Input: dimensioned drawing with shaded views. Units: mm. Origin: part minimum x, y, z. A direction names the side the tool comes from. Give positions to 0.01 mm unless a question says otherwise; leave off trailing zeros. Write each loop counter-clockwise with the first axis right and the second up, starting at its lowest first coordinate (ties: lowest second). Pieces come first, ordered by that corner, then holes.
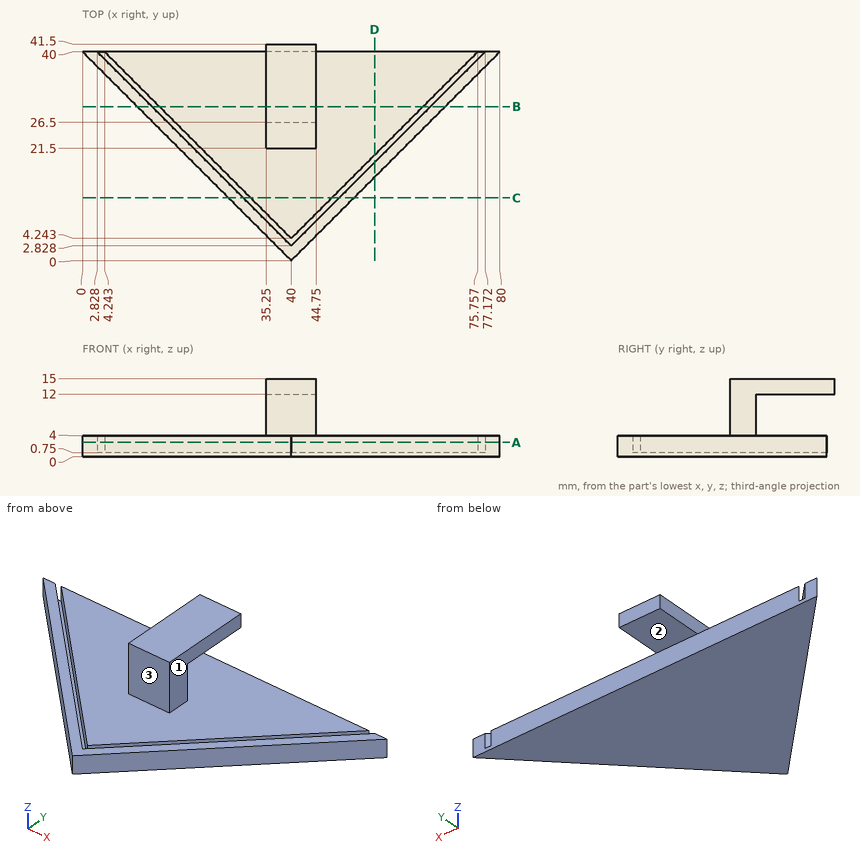
Item 1: Reachability of the marked faces 1, 2 and 3 from +Z, -Z, +X, -X, +Y, -Y: full face, straight path, thin tool, end or side. Return the list, or none.
Found:
face 1: +Z, +X, +Y, -Y
face 2: +X, -X, +Y
face 3: +Z, +X, -X, -Y
Item 2: Section B-B, the plane y = 29.5. Return the cut outline in (x, z), plus the area to 3 significant figures.
Found:
outline: (10.5, 0) - (69.5, 0) - (69.5, 4) - (66.67, 4) - (66.67, 0.75) - (65.26, 0.75) - (65.26, 4) - (14.74, 4) - (14.74, 0.75) - (13.33, 0.75) - (13.33, 4) - (10.5, 4) - close; (35.25, 12) - (44.75, 12) - (44.75, 15) - (35.25, 15) - close
area: 255 mm2
Item 3: Section A-A, the plane z = 2.75. Return the cut outline in (x, y).
Found:
outline: (0, 40) - (40, 0) - (80, 40) - (77.17, 40) - (40, 2.83) - (2.83, 40) - close; (4.24, 40) - (40, 4.24) - (75.76, 40) - close
Item 4: Section C-C, the plane y = 12. Return the cut outline in (x, z).
Found:
outline: (28, 0) - (52, 0) - (52, 4) - (49.17, 4) - (49.17, 0.75) - (47.76, 0.75) - (47.76, 4) - (32.24, 4) - (32.24, 0.75) - (30.83, 0.75) - (30.83, 4) - (28, 4) - close
Item 5: Section D-D, the plane x = 56. Return the cut outline in (y, z).
Found:
outline: (16, 0) - (40, 0) - (40, 4) - (20.24, 4) - (20.24, 0.75) - (18.83, 0.75) - (18.83, 4) - (16, 4) - close
Item 6: Pin query (flat end, axial travel): pin 1 Ø9 at (y, z) = (29, 9.5) entering from -X; pin 2 Ø3 at (x, y) = (22, 26) entering from +Z; pin 3 Ø6.5 at (x, z) = (39, 8) entering from +Y. Return the tip coordinate at first contact, or that it passes through.
Found:
pin 1: stops at x = 35.25
pin 2: stops at z = 4
pin 3: stops at y = 26.5
Item 7: Line query: L1, parallel to X at y = 32, z = 1.25 (1 decimal); L2, parallel to X at y = 24, z = 1.75 (1 decimal); L3, parallel to Z at x = 61, y = 35.5. Output: solid intervals per line, ascending.
Found:
L1: x = 8 to 10.8, 12.2 to 67.8, 69.2 to 72
L2: x = 16 to 18.8, 20.2 to 59.8, 61.2 to 64
L3: z = 0 to 4
